CAD build for the part. Positions are in the model's coordinates, mm. Give positions to 0.01 mm unless a question says otherwise; leave off trailing zeros. Loops run counter-clockwise (first coordinate to the right, second up) from the corner with the lowest first, then second, coordinate; pieces in that order, holes last. Notation, with made-up numbers: M 48,3 L 86,3 A24 cw 86,19 Z; hole C 75,48.5 d8. An arc over 180 degrees is marked long. Answer as CSV lines item,"result".
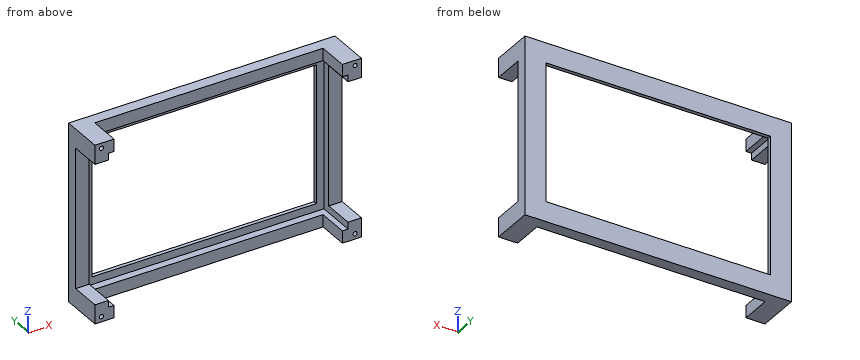
```python
from build123d import *

# Parameters (mm, degrees)
SKETCH1_W           = 177.165
SKETCH1_H           = 118.4275
SKETCH1_W_2         = 159.258
SKETCH1_H_2         = 102.108
BOSS_EXTRUDE1_DEPTH = 28.194
SKETCH2_W           = 159.258
SKETCH2_H           = 2.54
BOSS_EXTRUDE2_DEPTH = 5.08
SKETCH3_W           = 97.028
SKETCH3_H           = 2.54
BOSS_EXTRUDE3_DEPTH = 5.08
SKETCH4_W           = 154.178
SKETCH4_H           = 2.54
BOSS_EXTRUDE4_DEPTH = 5.08
SKETCH5_W           = 91.948
SKETCH5_H           = 2.54
BOSS_EXTRUDE5_DEPTH = 5.08
SKETCH10_W          = 93.0275
SKETCH10_H          = 20.574
CUT_EXTRUDE4_DEPTH  = 198.628
SKETCH9_W           = 151.765
SKETCH9_H           = 20.574
CUT_EXTRUDE5_DEPTH  = 198.628
SKETCH11_R          = 1.37795
CUT_EXTRUDE6_DEPTH  = 12.7


with BuildPart() as part:
    # Sketch1 → Boss-Extrude1 (new body)
    with BuildSketch(Plane(origin=(0, 0, 0), x_dir=(1, 0, 0), z_dir=(0, 1, 0))):
        with Locations((79.375, -50.8)):
            Rectangle(SKETCH1_W, SKETCH1_H)
        with Locations((79.375, -50.8)):
            Rectangle(SKETCH1_W_2, SKETCH1_H_2, mode=Mode.SUBTRACT)
    extrude(amount=-BOSS_EXTRUDE1_DEPTH)

    # Sketch2 → Boss-Extrude2 (add)
    with BuildSketch(Plane.XY.offset(-0.254)):
        with Locations((79.375, -1.27)):
            Rectangle(SKETCH2_W, SKETCH2_H)
    extrude(amount=BOSS_EXTRUDE2_DEPTH)

    # Sketch3 → Boss-Extrude3 (add)
    with BuildSketch(Plane(origin=(-0.254, 0, 0), x_dir=(0, 0, -1), z_dir=(1, 0, 0))):
        with Locations((-53.34, -1.27)):
            Rectangle(SKETCH3_W, SKETCH3_H)
    extrude(amount=BOSS_EXTRUDE3_DEPTH)

    # Sketch4 → Boss-Extrude4 (add)
    with BuildSketch(Plane(origin=(0, 0, 101.854), x_dir=(-1, 0, 0), z_dir=(0, 0, -1))):
        with Locations((-81.915, -1.27)):
            Rectangle(SKETCH4_W, SKETCH4_H)
    extrude(amount=BOSS_EXTRUDE4_DEPTH)

    # Sketch5 → Boss-Extrude5 (add)
    with BuildSketch(Plane.ZY.offset(-159.004)):
        with Locations((50.8, -1.27)):
            Rectangle(SKETCH5_W, SKETCH5_H)
    extrude(amount=BOSS_EXTRUDE5_DEPTH)

    # Sketch10 → Cut-Extrude4 (cut)
    with BuildSketch(Plane.ZY.offset(9.2075)):
        with Locations((50.8, -17.907)):
            Rectangle(SKETCH10_W, SKETCH10_H)
    extrude(amount=-CUT_EXTRUDE4_DEPTH, mode=Mode.SUBTRACT)

    # Sketch9 → Cut-Extrude5 (cut)
    with BuildSketch(Plane.XY.offset(110.01375)):
        with Locations((79.375, -17.907)):
            Rectangle(SKETCH9_W, SKETCH9_H)
    extrude(amount=-CUT_EXTRUDE5_DEPTH, mode=Mode.SUBTRACT)

    # Sketch11 → Cut-Extrude6 (cut)
    with BuildSketch(Plane.XZ.offset(28.194)):
        with Locations((-4.8895, 106.58475)):
            Circle(SKETCH11_R)
        with Locations((-4.8895, -4.92125)):
            Circle(SKETCH11_R)
        with Locations((163.7665, -4.92125)):
            Circle(SKETCH11_R)
        with Locations((163.7665, 106.58475)):
            Circle(SKETCH11_R)
    extrude(amount=-CUT_EXTRUDE6_DEPTH, mode=Mode.SUBTRACT)


solid = part.part
```
Q1. Pin check, flat tips, straight feed: P1, Ø3, axis at x = -5, z = 107, coming from the -Y side; P2, Ø2, axis at x = 163.77, z = 106.58, coming from the -Y side. Stop position of each tip, or through.
Solution:
P1,"stops at y = -28.19"
P2,"stops at y = -15.49"
Q2. Cut at C-C (x = 41.5). Write the cut outline in (y, z).
Solution:
outline,"M -7.62,-8.41 L 0,-8.41 L 0,4.83 L -2.54,4.83 L -2.54,-0.25 L -7.62,-0.25 Z; M -7.62,101.85 L -2.54,101.85 L -2.54,96.77 L 0,96.77 L 0,110.01 L -7.62,110.01 Z"
Q3. Cut at D-D (y = -13.5). Write the cut outline in (x, z), and give its area (3 significant figures).
Solution:
outline,"M -9.21,-8.41 L 3.49,-8.41 L 3.49,-0.25 L -0.25,-0.25 L -0.25,4.29 L -9.21,4.29 Z; M -9.21,97.31 L -0.25,97.31 L -0.25,101.85 L 3.49,101.85 L 3.49,110.01 L -9.21,110.01 Z; M 155.26,-8.41 L 167.96,-8.41 L 167.96,4.29 L 159,4.29 L 159,-0.25 L 155.26,-0.25 Z; M 155.26,101.85 L 159,101.85 L 159,97.31 L 167.96,97.31 L 167.96,110.01 L 155.26,110.01 Z"
area,"577 mm²"
Q4. Wall check: line 1 (Z direction, x = 94, y = -7.25); line 2 (X direction, y = -4.5, z = 83.5); line 3 (X direction, y = -16.75, z = -2). Give the ranges that are in metal, low to high. Write a range as [from, to].
Solution:
line 1,"z = [-8.41, -0.25], [101.85, 110.01]"
line 2,"x = [-9.21, -0.25], [159, 167.96]"
line 3,"x = [-9.21, 3.49], [155.26, 167.96]"
Q5. Cut at B-B (y = -26). Write the cut outline in (x, z), and give its area (3 significant figures).
Solution:
outline,"M -9.21,-8.41 L 3.49,-8.41 L 3.49,-0.25 L -0.25,-0.25 L -0.25,4.29 L -9.21,4.29 Z; M -9.21,97.31 L -0.25,97.31 L -0.25,101.85 L 3.49,101.85 L 3.49,110.01 L -9.21,110.01 Z; M 155.26,-8.41 L 167.96,-8.41 L 167.96,4.29 L 159,4.29 L 159,-0.25 L 155.26,-0.25 Z; M 155.26,101.85 L 159,101.85 L 159,97.31 L 167.96,97.31 L 167.96,110.01 L 155.26,110.01 Z; hole C -4.89,-4.92 d2.76; hole C -4.89,106.58 d2.76; hole C 163.77,-4.92 d2.76; hole C 163.77,106.58 d2.76"
area,"553 mm²"
Q6. Cut at A-A (z = 78.5). Write the cut outline in (x, y).
Solution:
outline,"M -9.21,-7.62 L -0.25,-7.62 L -0.25,-2.54 L 4.83,-2.54 L 4.83,0 L -9.21,0 Z; M 153.92,-2.54 L 159,-2.54 L 159,-7.62 L 167.96,-7.62 L 167.96,0 L 153.92,0 Z"
